Here's how the part is built. I have some questions about the finished solid (model axes, mm). A direction names the side the tool comes from. Round coordinates to 2 decimals unless told otherwise and drop trailing zeros. Order: outer loops, then holes, each group sorted by start corner. A loop starts at its lowest first (then second) coordinate and runs counter-clockwise, first axis right, second up. Notation, with made-up numbers: (31, -27.5) - (55, -27.5) arc R13 cw to (55, -20.5) - close; hole circle Ø8 at (68, 20.25). An arc over 180 degrees is marked (long way). Answer as a JSON object with one key per item and string values.
```python
from build123d import *

# Parameters (mm, degrees)
CYLINDER020_R             = 11.1
CYLINDER020_DEPTH         = 26
CYLINDER019_R             = 4
CYLINDER019_DEPTH         = 43
CYLINDER021_R             = 1
CYLINDER021_DEPTH         = 31
CYLINDER024_R             = 1
CYLINDER024_DEPTH         = 31
CYLINDER023_R             = 1
CYLINDER023_DEPTH         = 31
CYLINDER022_R             = 1
CYLINDER022_DEPTH         = 31
FUSION002_ROLL_ANGLE      = -90
FUSION003_PLACEMENT_ANGLE = 180
SKETCH_R                  = 5
SKETCH_R_2                = 1.75
PAD_DEPTH                 = 6
CUT_PITCH_ANGLE           = 90


with BuildPart() as cylinder141:
    # Cylinder020 → Cylinder020 (new body)
    with BuildSketch(Plane(origin=(-3, 71, 73), x_dir=(0, 0, 1), z_dir=(0, -1, 0))):
        Circle(CYLINDER020_R)
    extrude(amount=CYLINDER020_DEPTH)


with BuildPart() as fusion001:
    # Cylinder019 → Cylinder019 (new body)
    with BuildSketch(Plane(origin=(-3, 66, 73), x_dir=(0, 0, 1), z_dir=(0, -1, 0))):
        Circle(CYLINDER019_R)
    extrude(amount=CYLINDER019_DEPTH)

    # Fusion001: union Cylinder141
    add(cylinder141.part)


with BuildPart() as cylinder096:
    # Cylinder021 → Cylinder021 (new body)
    with BuildSketch(Plane(origin=(-7.5, -11, 132), x_dir=(1, 0, 0), z_dir=(0, 0, 1))):
        Circle(CYLINDER021_R)
    extrude(amount=CYLINDER021_DEPTH)


with BuildPart() as cylinder146:
    # Cylinder024 → Cylinder024 (new body)
    with BuildSketch(Plane(origin=(0, -3.5, 132), x_dir=(1, 0, 0), z_dir=(0, 0, 1))):
        Circle(CYLINDER024_R)
    extrude(amount=CYLINDER024_DEPTH)


with BuildPart() as cylinder145:
    # Cylinder023 → Cylinder023 (new body)
    with BuildSketch(Plane(origin=(7.5, -11, 132), x_dir=(1, 0, 0), z_dir=(0, 0, 1))):
        Circle(CYLINDER023_R)
    extrude(amount=CYLINDER023_DEPTH)


with BuildPart() as fusion003:
    # Cylinder022 → Cylinder022 (new body)
    with BuildSketch(Plane(origin=(0, -18.5, 132), x_dir=(1, 0, 0), z_dir=(0, 0, 1))):
        Circle(CYLINDER022_R)
    extrude(amount=CYLINDER022_DEPTH)

    # Fusion002: union Cylinder096, Cylinder146, Cylinder145
    add(cylinder096.part)
    add(cylinder146.part)
    add(cylinder145.part)


with BuildPart() as fusion003_1:
    # Fusion002 roll: moved
    add(fusion003.part.rotate(Axis((0, 0, 0), (1, 0, 0)), FUSION002_ROLL_ANGLE))


with BuildPart() as fusion003_2:
    # Fusion002 placement: moved
    add(fusion003_1.part.moved(Location((-3, -97.5, 62))))

    # Fusion003: union Fusion001
    add(fusion001.part)


with BuildPart() as fusion003_3:
    # Fusion003 placement: moved
    add(fusion003_2.part.moved(Location((-0.5, 88, -87))).rotate(Axis((-0.5, 88, -87), (0, 0, 1)), FUSION003_PLACEMENT_ANGLE))


with BuildPart() as clone_of_cut:
    # Sketch → Pad (new body)
    with BuildSketch(Plane(origin=(-11.5, 40, -16.5), x_dir=(0, 0, -1), z_dir=(0, 1, 0))):
        with BuildLine():
            Line((-2.5, -3), (47.5, -3))
            ThreePointArc((47.5, -25), (58.5, -14), (47.5, -3))
            Line((-2.5, -25), (47.5, -25))
            ThreePointArc((-2.5, -3), (-13.5, -14), (-2.5, -25))
        make_face()
        with Locations((14.166667, -14)):
            Circle(SKETCH_R, mode=Mode.SUBTRACT)
        with Locations((30.833333, -14)):
            Circle(SKETCH_R, mode=Mode.SUBTRACT)
        with Locations((47.5, -14)):
            Circle(SKETCH_R_2, mode=Mode.SUBTRACT)
    extrude(amount=PAD_DEPTH)

    # Cut: cut Fusion003
    add(fusion003_3.part, mode=Mode.SUBTRACT)


with BuildPart() as clone_of_cut_1:
    # Cut pitch: moved
    add(clone_of_cut.part.rotate(Axis((0, 0, 0), (0, 1, 0)), CUT_PITCH_ANGLE))


with BuildPart() as clone_of_cut_2:
    # Cut placement: moved
    add(clone_of_cut_1.part.moved(Location((16.5, -87, -15))))


with BuildPart() as clone_of_cut_3:
    # Clone010 placement: moved
    add(clone_of_cut_2.part.moved(Location((0, 0, -22.5))))


with BuildPart() as part_mirroring026:
    # Part__Mirroring026: instance of Clone of Cut
    add(clone_of_cut_3.part.mirror(Plane(origin=(0, 0, 0), x_dir=(1, 0, 0), z_dir=(0, 1, 0))))


solid = part_mirroring026.part
```
1. Imagine slicing it at B-B (y = 44.75). List the corners of the cut face in (x, z) for me, plus the area to 3 significant figures.
Responses:
{"outline": "(-47.5, -51) - (1.01, -51) arc R11.1 cw to (1.01, -29) - (-47.5, -29) arc R11 ccw to start; hole circle Ø3.5 at (-47.5, -40); hole circle Ø10 at (-30.83, -40); hole circle Ø10 at (-14.17, -40)", "area": "930 mm2"}
2. Imagine slicing it at C-C (x = 10). List the corners of the cut face in (y, z) for me.
Responses:
{"outline": "(41, -48.05) - (44, -48.05) - (44, -41) - (41, -41) - close; (41, -39) - (44, -39) - (44, -31.95) - (41, -31.95) - close"}
3. If I drill on L1, parallel to Z at x = -7.5, y = 45.25; L2, parallel to Z at x = -47.5, y = 44.75; L3, parallel to Y at x = 8.5, z = -38.25, over which ranges is the centre line in solid material (lowest first)? Write a range as [from, to].
Responses:
{"L1": "[-51, -44.82], [-35.18, -29]", "L2": "[-51, -41.75], [-38.25, -29]", "L3": "[41, 44]"}
4. Thinking about a two-plate mould opening in X: for faces 3 (the face through (-36, 47, -37)), 4 (the face through (13.5, 42.5, -39.8)), 5 (the face through (2.2, 42.479, -46.546)), which applies, pulls with the +X half, pulls with the -X half, needs draft (parallel to the pull), parting line crosses it, or undercut?
Responses:
{"face 3": "needs draft", "face 4": "pulls with the +X half", "face 5": "undercut"}
5. Imagine slicing it at D-D (z = -47.5). List the corners of the cut face in (x, y) for me, plus the area to 3 significant figures.
Responses:
{"outline": "(-55.55, 41) - (1.5, 41) - (1.5, 44) - (-5.68, 44) - (-5.68, 47) - (-55.55, 47) - close; (3.5, 41) - (10.55, 41) - (10.55, 44) - (3.5, 44) - close", "area": "342 mm2"}
6. Imagine slicing it at A-A (z = -40). Give the number of separate pieces and of enclosed holes in the cut face, plus the area to 3 significant figures.
Responses:
{"separate pieces": "7", "enclosed holes": "0", "area": "189 mm2"}
7. For faces 1 (the face through (-22, 44, -51)), 2 (the face through (2, 44, -35)), which set-ups out of +Z, -Z, +X, -X, +Y, -Y let a thin tool reach every point of the face, with its end or its side?
Responses:
{"face 1": "-Z, +X, -X, +Y, -Y", "face 2": "+X, +Y"}
8. For P1, Ø2, axis at x = 2, y = 44.5, coming from the +Z side; P2, Ø3, axis at x = 10, z = -40, coming from the +Y side; P3, Ø3, axis at y = 45.5, z = -34, coming from the -X side; P4, Ø7, axis at x = 2.5, z = -40, coming from the +Y side (3 decimals), each with a flat end and sliding along its axis, tell me the tip position at first contact or that it passes through.
Responses:
{"P1": "z = -29", "P2": "y = 44", "P3": "x = -57.54", "P4": "through"}
